from build123d import *

# Parameters (mm, degrees)
NECK_DEPTH = 10.9728


# Read off the part's stored shape, not the designer's step: Cut-Revolve1
with BuildPart() as part:
    # Cut-Revolve1 outline → Cut-Revolve1 (revolve)
    with BuildSketch(Plane.YX):
        Polygon((0, 76.2), (0, 0), (11.6459, 0), (11.6459, 0.533667773), (4.7625, 5.0038), (4.7625, 76.2), align=None)
    revolve(axis=Axis((0, 0, 0), (1, 0, 0)))

    # Sketch2 → Neck (add)
    with BuildSketch(Plane(origin=(0, 0, 0), x_dir=(0, 0.6946583704589985, -0.7193398003386501), z_dir=(1, 0, 0))):
        with BuildLine():
            Line((3.5687, -4.7625), (-3.5687, -4.7625))
            ThreePointArc((-3.5687, -4.7625), (-4.412844075, -4.412844075), (-4.7625, -3.5687))
            Line((-4.7625, -3.5687), (-4.7625, 3.5687))
            ThreePointArc((-4.7625, 3.5687), (-4.412844075, 4.412844075), (-3.5687, 4.7625))
            Line((-3.5687, 4.7625), (3.5687, 4.7625))
            ThreePointArc((3.5687, 4.7625), (4.412844075, 4.412844075), (4.7625, 3.5687))
            Line((4.7625, 3.5687), (4.7625, -3.5687))
            ThreePointArc((4.7625, -3.5687), (4.412844075, -4.412844075), (3.5687, -4.7625))
        make_face()
    extrude(amount=NECK_DEPTH)


solid = part.part
Here's how the part is built. I have some questions about the finished solid (model axes, mm). A direction names the side the tool comes from. Give positions to 0.01 mm unless a question says otherwise; leave off trailing zeros. Order: outer loops, then holes, each group sorted by start corner. A loop starts at its lowest first (then second) coordinate and runs counter-clockwise, first axis right, second up. Notation, with made-up numbers: (23, -25) -> (62, -25) arc R19 ccw to (62, 3) -> close; hole circle Ø1 at (40.5, -21). An arc over 180 degrees is marked (long way). Use a Markdown table: item, result. Add a question column.
Item 1: I need wall thicknesses on line 1 (X direction, y = 6.5, z = 9.25); line 2 (X direction, y = 1, z = 5.5); line 3 (Z direction, x = 12, y = 2). Which ranges of each line are inside material? Lowest first, please.
Item 2: Imagine slicing it at A-A on z = 0. Please give me the cut outline in (x, y).
Item 3: For faces 1 (the face through (7.555, -3.391, -3.344)), 2 (the face through (7.555, -3.344, 3.391)), 3 (the face through (7.46, -6.24, 0.1)), which set-ups out of +Z, -Z, +X, -X, +Y, -Y let a thin tool reach every point of the face, with its end or its side?
Item 4: Imagine slicing it at B-B on x = 53.5. Please give me the cut outline in (y, z) (1 decimal), plus the area to 3 significant figures.
Item 5: Will these pins go through, and if not, where does the flat tip stop? pin 1 (12 mm diameter, centred on y = -4, z = -8, fed in from +X); pin 2 (8 mm diameter, centred on x = 30.5, z = 2.5, fed in from -Y); pin 3 (4 mm diameter, centred on x = 22, y = 5, fed in from -Z); pin 4 (10 mm diameter, centred on x = 52.5, y = 1.5, fed in from -Z).
Data:
| question | item | result |
|---|---|---|
| 1 | line 1 | x = 0 to 0.75 |
| 1 | line 2 | x = 0 to 10.97 |
| 1 | line 3 | z = -4.32 to 4.32 |
| 2 | outline | (0, -11.65) -> (0.53, -11.65) -> (4.05, -6.24) -> (10.97, -6.24) -> (10.97, -4.76) -> (76.2, -4.76) -> (76.2, 4.76) -> (10.97, 4.76) -> (10.97, 6.24) -> (4.05, 6.24) -> (0.53, 11.65) -> (0, 11.65) -> close |
| 3 | face 1 | -Z, +X, -Y |
| 3 | face 2 | +Z, +X, -Y |
| 3 | face 3 | +X, -Y |
| 4 | outline | circle Ø9.5 at (0, 0) |
| 4 | area | 71.3 mm² |
| 5 | pin 1 | stops at x = 76.2 |
| 5 | pin 2 | stops at y = -4.76 |
| 5 | pin 3 | stops at z = -3.7 |
| 5 | pin 4 | stops at z = -4.76 |
